Input: part model. Units: mm. Frame: model coordinates. Face numbers are marked on the shaded views. A direction names the side the tool comes from. Coordinates: 2 decimals unless noted, no trailing zeros. Order: outer loops, then holes, each group sorted by start corner. A loop starts at its lowest first (then second) coordinate and runs counter-clockwise, first axis right, second up. Notation, with made-up numbers: (28, 50) - (70, 50) arc R18 cw to (70, 59) - close; hole circle Ø5 at (-15, -17.75). An arc over 180 degrees is marked (long way). One line per question, with ' | ' between items. Start each with the question number.
```python
from build123d import *

# Parameters (mm, degrees)
BASE_FLANGIA1_DEPTH                  = 3.5
PIEGATURA_START                      = -30
PIEGATURA_DELLO_SCHIZZO1_DEPTH       = 60
PIEGATURA_DELLO_SCHIZZO1_2_OUTLINE_W = 3.5
PIEGATURA_DELLO_SCHIZZO1_2_OUTLINE_H = 9.495553214
PIEGATURA_DELLO_SCHIZZO1_2_DEPTH     = 60
FORO_PER_VITE_M4_1_D                 = 4.3
FORO_PER_VITE_M4_1_DEPTH             = 20
FORO_PER_VITE_M4_1_TIP               = 1.291850331
FORO_PER_VITE_M3_1_AT_2_COUNT        = 2
FORO_PER_VITE_M3_1_AT_2_PITCH        = 48
FORO_PER_VITE_M3_1_AT_3_COUNT        = 2
FORO_PER_VITE_M3_1_AT_3_PITCH        = 60
FORO_PER_VITE_M3_1_AT_4_COUNT        = 2
FORO_PER_VITE_M3_1_AT_4_PITCH        = 36
RIPETIZIONE_A_L1_COUNT               = 2
RIPETIZIONE_A_L1_PITCH               = 60
RIPETIZIONE_A_L1_COL_COUNT           = 2
RIPETIZIONE_A_L1_COL_PITCH           = 60


# Read off the part's stored shape, not the designer's step: Piegatura dello schizzo1
# Sheet-metal steps are written as plain solids
with BuildPart() as part:
    # Schizzo1 → Base-Flangia1 (new body)
    with BuildSketch(Plane.XY):
        Polygon((-45, 95), (45, 95), (45, 30), (94, 30), (94, -30), (45, -30), (45, -95), (-45, -95), align=None)
    extrude(amount=-BASE_FLANGIA1_DEPTH)

    # Piegatura dello schizzo1 outline → Piegatura dello schizzo1 (cut)
    with BuildSketch(Plane(origin=(0, 0, 0), x_dir=(1, 0, 0), z_dir=(0, 1, 0)).offset(PIEGATURA_START)):
        with BuildLine():
            Line((94, 3.5), (85.255553214, 3.5))
            ThreePointArc((85.255553214, 3.5), (84.230426948, 1.025126266), (81.755553214, 0))
            Line((81.755553214, 0), (94, 0))
            Line((94, 0), (94, 3.5))
        make_face()
    extrude(amount=PIEGATURA_DELLO_SCHIZZO1_DEPTH, mode=Mode.SUBTRACT)

    # Piegatura dello schizzo1 2 outline → Piegatura dello schizzo1 2 (add)
    with BuildSketch(Plane(origin=(0, 0, 0), x_dir=(1, 0, 0), z_dir=(0, 1, 0)).offset(PIEGATURA_START)):
        with Locations((83.505553214, 8.247776607)):
            Rectangle(PIEGATURA_DELLO_SCHIZZO1_2_OUTLINE_W, PIEGATURA_DELLO_SCHIZZO1_2_OUTLINE_H)
    extrude(amount=PIEGATURA_DELLO_SCHIZZO1_2_DEPTH)

    # Foro per Vite M4-1
    with Locations(Plane(origin=(76, 24, 0), x_dir=(1, 0, 0), z_dir=(0, 0, 1))):
        with Locations((0, 0), (0, -48)):
            Hole(FORO_PER_VITE_M4_1_D / 2, depth=FORO_PER_VITE_M4_1_DEPTH)
            with Locations((0, 0, -(FORO_PER_VITE_M4_1_DEPTH + FORO_PER_VITE_M4_1_TIP / 2))):  # 118° drill point
                Cone(0, FORO_PER_VITE_M4_1_D / 2, FORO_PER_VITE_M4_1_TIP, mode=Mode.SUBTRACT)

    # Schizzo9 → Foro per Vite M3-1 (revolve, cut)
    with BuildSketch(Plane(origin=(-28, 24, 0), x_dir=(0, -1, 0), z_dir=(1, 0, 0))):
        Polygon((0, 0), (0, 20.96137699), (1.6, 20), (1.6, 0), align=None)
    foro_per_vite_m3_1 = revolve(axis=Axis((-28, 24, 6.35), (0, 0, -1)), mode=Mode.SUBTRACT)

    # Foro per Vite M3-1 at 2: Foro per Vite M3-1 ×2
    with Locations(*[(0, -i * FORO_PER_VITE_M3_1_AT_2_PITCH, 0) for i in range(1, FORO_PER_VITE_M3_1_AT_2_COUNT)]):
        add(foro_per_vite_m3_1, mode=Mode.SUBTRACT)

    # Foro per Vite M3-1 at 3: Foro per Vite M3-1 ×2
    with Locations(*[Vector(0.6000000000000001, -0.7999999999999999, 0) * (i * FORO_PER_VITE_M3_1_AT_3_PITCH) for i in range(1, FORO_PER_VITE_M3_1_AT_3_COUNT)]):
        add(foro_per_vite_m3_1, mode=Mode.SUBTRACT)

    # Foro per Vite M3-1 at 4: Foro per Vite M3-1 ×2
    with Locations(*[(i * FORO_PER_VITE_M3_1_AT_4_PITCH, 0, 0) for i in range(1, FORO_PER_VITE_M3_1_AT_4_COUNT)]):
        add(foro_per_vite_m3_1, mode=Mode.SUBTRACT)

    # Ripetizione a L1: Foro per Vite M3-1 ×2
    with Locations(*[(0, -i * RIPETIZIONE_A_L1_PITCH, 0) for i in range(1, RIPETIZIONE_A_L1_COUNT)]):
        add(foro_per_vite_m3_1, mode=Mode.SUBTRACT)

    # Ripetizione a L1 copy 1 sketch → Ripetizione a L1 copy 1 (revolve, cut)
    with BuildSketch(Plane(origin=(-28, -84, 0), x_dir=(0, -1, 0), z_dir=(1, 0, 0))):
        Polygon((0, 0), (0, 20.96137699), (1.6, 20), (1.6, 0), align=None)
    revolve(axis=Axis((-28, -84, 6.35), (0, 0, -1)), mode=Mode.SUBTRACT)

    # Ripetizione a L1 copy 2 sketch → Ripetizione a L1 copy 2 (revolve, cut)
    with BuildSketch(Plane(origin=(8, -84, 0), x_dir=(0, -1, 0), z_dir=(1, 0, 0))):
        Polygon((0, 0), (0, 20.96137699), (1.6, 20), (1.6, 0), align=None)
    revolve(axis=Axis((8, -84, 6.35), (0, 0, -1)), mode=Mode.SUBTRACT)

    # Ripetizione a L1 copy 3 sketch → Ripetizione a L1 copy 3 (revolve, cut)
    with BuildSketch(Plane(origin=(8, -36, 0), x_dir=(0, -1, 0), z_dir=(1, 0, 0))):
        Polygon((0, 0), (0, 20.96137699), (1.6, 20), (1.6, 0), align=None)
    revolve(axis=Axis((8, -36, 6.35), (0, 0, -1)), mode=Mode.SUBTRACT)

    # Ripetizione a L1 col: Foro per Vite M3-1 ×2
    with Locations(*[(0, i * RIPETIZIONE_A_L1_COL_PITCH, 0) for i in range(1, RIPETIZIONE_A_L1_COL_COUNT)]):
        add(foro_per_vite_m3_1, mode=Mode.SUBTRACT)

    # Ripetizione a L1 col copy 1 sketch → Ripetizione a L1 col copy 1 (revolve, cut)
    with BuildSketch(Plane(origin=(-28, 36, 0), x_dir=(0, -1, 0), z_dir=(1, 0, 0))):
        Polygon((0, 0), (0, 20.96137699), (1.6, 20), (1.6, 0), align=None)
    revolve(axis=Axis((-28, 36, 6.35), (0, 0, -1)), mode=Mode.SUBTRACT)

    # Ripetizione a L1 col copy 2 sketch → Ripetizione a L1 col copy 2 (revolve, cut)
    with BuildSketch(Plane(origin=(8, 36, 0), x_dir=(0, -1, 0), z_dir=(1, 0, 0))):
        Polygon((0, 0), (0, 20.96137699), (1.6, 20), (1.6, 0), align=None)
    revolve(axis=Axis((8, 36, 6.35), (0, 0, -1)), mode=Mode.SUBTRACT)

    # Ripetizione a L1 col copy 3 sketch → Ripetizione a L1 col copy 3 (revolve, cut)
    with BuildSketch(Plane(origin=(8, 84, 0), x_dir=(0, -1, 0), z_dir=(1, 0, 0))):
        Polygon((0, 0), (0, 20.96137699), (1.6, 20), (1.6, 0), align=None)
    revolve(axis=Axis((8, 84, 6.35), (0, 0, -1)), mode=Mode.SUBTRACT)


solid = part.part
```
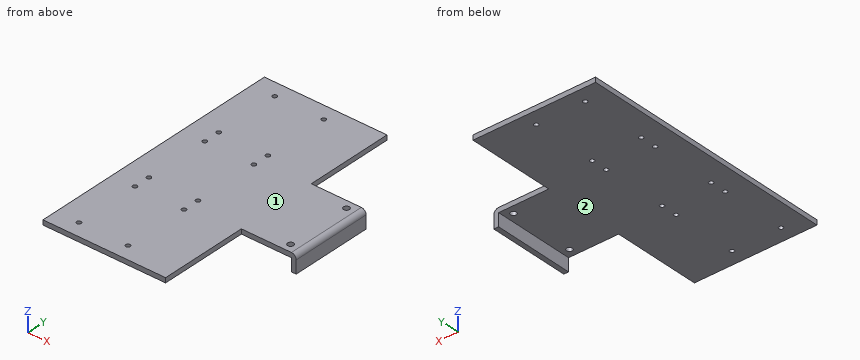
(1) Section C-C (z = -10.5). Output: boundary loops of the cut face in (x, y), then the cut area to 3 significant figures.
(2) Pin query (flat end, axial travel): pin 1 (6 mm diameter, centred on x = 33.5, y = 73.5, fed in from -Z); pin 2 (2.5 mm diameter, centred on x = 76, y = 24, fed in from +Z); pin 3 (4 mm diameter, centred on y = 72.5, z = -1.5, fed in from +X). Return the tip coordinate at first contact, or that it passes through.
(3) Section B-B (y = -6.5). Output: boundary loops of the cut face in (x, z).
(4) Section A-A (x = 76). Output: boundary loops of the cut face in (y, z).
(5) Section D-D (x = -10.5). Output: boundary loops of the cut face in (y, z).
(6) Reachability of the marked faces 1 and 2 from +Z, -Z, +X, -X, +Y, -Y: full face, straight path, thin tool, end or side. Return the list, or none.
(7) Material intervals for line 1 along X through (y, z) = (84, -0.9); line 2 along Z through (x, y) = (23, 64.5); line 3 along X through (y, z) = (5.5, -5.75), sorted ascending. Write a range as from..to.
Worked answers:
1) outline: (81.76, -30) - (85.26, -30) - (85.26, 30) - (81.76, 30) - close | area: 210 mm²
2) pin 1: stops at z = -3.5 | pin 2: passes through | pin 3: stops at x = 45
3) outline: (-45, -3.5) - (81.76, -3.5) - (81.76, -13) - (85.26, -13) - (85.26, -3.5) arc R3.5 ccw to (81.76, 0) - (-45, 0) - close
4) outline: (-30, -3.5) - (-26.15, -3.5) - (-26.15, 0) - (-30, 0) - close; (-21.85, -3.5) - (21.85, -3.5) - (21.85, 0) - (-21.85, 0) - close; (26.15, -3.5) - (30, -3.5) - (30, 0) - (26.15, 0) - close
5) outline: (-95, -3.5) - (95, -3.5) - (95, 0) - (-95, 0) - close
6) face 1: +Z, +X, -X, +Y, -Y | face 2: -Z, -X, +Y, -Y
7) line 1: x = -45..-29.6, -26.4..6.4, 9.6..45 | line 2: z = -3.5..0 | line 3: x = 81.76..85.26
